For this review, take the finished solid that the model builds, in its own axes (mm). A direction names the side the tool comes from. Coordinates: 2 decimals unless noted, no trailing zeros. Loops run counter-clockwise (first coordinate to the right, second up) from the corner with the lowest first, then second, coordinate; pieces in that order, holes last. Notation, with made-up numbers: M 20,9 L 63,9 A20 ccw 63,41 Z; hole C 14.5,31 d9. An arc over 180 degrees is marked long. Write each question's results on one line, items separated by ' | '. Start each with the question number.
```python
from build123d import *

# Parameters (mm, degrees)
SKETCH1_R           = 80
BOSS_EXTRUDE1_DEPTH = 3.5
SKETCH2_R           = 10
CUT_EXTRUDE1_DEPTH  = 3.5
BOSS_EXTRUDE2_START = 10
SKETCH3_R           = 30
SKETCH3_R_2         = 10
BOSS_EXTRUDE2_DEPTH = 10
CUT_EXTRUDE2_DEPTH  = 3.5


with BuildPart() as part:
    # Sketch1 → Boss-Extrude1 (new body)
    with BuildSketch(Plane.XY):
        Circle(SKETCH1_R)
    extrude(amount=BOSS_EXTRUDE1_DEPTH)

    # Sketch2 → Cut-Extrude1 (cut)
    with BuildSketch(Plane.XY.offset(3.5)):
        Circle(SKETCH2_R)
    extrude(amount=-CUT_EXTRUDE1_DEPTH, mode=Mode.SUBTRACT)

    # Sketch3 → Boss-Extrude2 (add)
    with BuildSketch(Plane.XY.offset(3.5).offset(BOSS_EXTRUDE2_START)):
        Circle(SKETCH3_R)
        Circle(SKETCH3_R_2, mode=Mode.SUBTRACT)
    extrude(amount=-BOSS_EXTRUDE2_DEPTH)

    # Sketch6 → Cut-Extrude2 (cut)
    with BuildSketch(Plane.XY.offset(3.5)):
        with BuildLine():
            Line((36.837168574, 28.196152423), (51.559600438, 36.696152423))
            ThreePointArc((51.559600438, 36.696152423), (59.755752861, 34.5), (57.559600438, 26.303847577))
            Line((57.559600438, 26.303847577), (42.837168574, 17.803847577))
            ThreePointArc((42.837168574, 17.803847577), (34.641016151, 20), (36.837168574, 28.196152423))
        make_face()
        with BuildLine():
            Line((42.837168574, -17.803847577), (57.559600438, -26.303847577))
            ThreePointArc((57.559600438, -26.303847577), (59.755752861, -34.5), (51.559600438, -36.696152423))
            Line((51.559600438, -36.696152423), (36.837168574, -28.196152423))
            ThreePointArc((36.837168574, -28.196152423), (34.641016151, -20), (42.837168574, -17.803847577))
        make_face()
        with BuildLine():
            Line((6, -46), (6, -63))
            ThreePointArc((6, -63), (0, -69), (-6, -63))
            Line((-6, -63), (-6, -46))
            ThreePointArc((-6, -46), (0, -40), (6, -46))
        make_face()
        with BuildLine():
            Line((-36.837168574, -28.196152423), (-51.559600438, -36.696152423))
            ThreePointArc((-51.559600438, -36.696152423), (-59.755752861, -34.5), (-57.559600438, -26.303847577))
            Line((-57.559600438, -26.303847577), (-42.837168574, -17.803847577))
            ThreePointArc((-42.837168574, -17.803847577), (-34.641016151, -20), (-36.837168574, -28.196152423))
        make_face()
        with BuildLine():
            Line((-42.837168574, 17.803847577), (-57.559600438, 26.303847577))
            ThreePointArc((-57.559600438, 26.303847577), (-59.755752861, 34.5), (-51.559600438, 36.696152423))
            Line((-51.559600438, 36.696152423), (-36.837168574, 28.196152423))
            ThreePointArc((-36.837168574, 28.196152423), (-34.641016151, 20), (-42.837168574, 17.803847577))
        make_face()
        with BuildLine():
            Line((-6, 46), (-6, 63))
            ThreePointArc((-6, 63), (0, 69), (6, 63))
            Line((6, 63), (6, 46))
            ThreePointArc((6, 46), (0, 40), (-6, 46))
        make_face()
    extrude(amount=-CUT_EXTRUDE2_DEPTH, mode=Mode.SUBTRACT)


solid = part.part
```
Q1. Insertion check: P1, Ø3, axis at y = -56, z = 1, coming from the +X side; P2, Ø1.8, axis at y = 52.5, z = 1, coming from the -X side; P3, Ø4, axis at x = -45.5, y = -13, coming from the +Z side. Each pin has a flat end and moves straight along its axis. Give the tip position at first contact, or say it passes through.
Q2. The part is to be moulded in two halves that separate along Y. For faces 1 (the face through (34, 1, 3.5)), 2 (the face through (50.301, 22.113, 1.774)), 3 (the face through (-17.34, -78.1, 1.73)), say which applies: pulls with the +Y half, pulls with the -Y half, needs draft (parallel to the pull), parting line crosses it, or undercut.
Q3. To check wall thickness, follow line 1 along Y through (x, z) = (0, 4); line 2 along Y through (x, z) = (-5, 3); line 3 along Z through (x, y) = (-39, 46). State the ranges of each line that lie inside material, in increasing order.
Q4. Take a section at B-B, the plane x = -0.5. Give the boundary of the cut face in (y, z).
Q5. Take a section at D-D, the plane x = 46.5. Give the boundary of the cut face in (y, z) (3 decimals), then the cut area to 3 significant figures.
Q6. Take a section at C-C, the plane y = 23. Give the boundary of the cut face in (x, z).
Q7. For faces 4 (the face through (-29.97, 1.32, 8.57)), 5 (the face through (13, 0, 13.5)), 6 (the face through (-6, 54, 2)), list the 3-axis set-ups (+Z, -Z, +X, -X, +Y, -Y) from which the entire face can be reached by the end or side of a thin tool; tool diameter is ignored.
Q8. Take a section at A-A, the plane y = 0. Give the boundary of the cut face in (x, z).
Results:
1) P1: x = 58.56 | P2: x = -61.13 | P3: z = 3.5
2) face 1: needs draft | face 2: undercut | face 3: parting line crosses it
3) line 1: -30 to -10, 10 to 30 | line 2: -79.84 to -66.32, -42.68 to -8.66, 8.66 to 42.68, 66.32 to 79.84 | line 3: 0 to 3.5
4) outline: M -80,0 L -68.98,0 L -68.98,3.5 L -80,3.5 Z; M -40.02,0 L -9.99,0 L -9.99,13.5 L -30,13.5 L -30,3.5 L -40.02,3.5 Z; M 9.99,0 L 40.02,0 L 40.02,3.5 L 30,3.5 L 30,13.5 L 9.99,13.5 Z; M 68.98,0 L 80,0 L 80,3.5 L 68.98,3.5 Z
5) outline: M -65.098,0 L -33.775,0 L -33.775,3.5 L -65.098,3.5 Z; M -19.919,0 L 19.919,0 L 19.919,3.5 L -19.919,3.5 Z; M 33.775,0 L 65.098,0 L 65.098,3.5 L 33.775,3.5 Z | area: 359 mm^2
6) outline: M -76.62,0 L -51.84,0 L -51.84,3.5 L -76.62,3.5 Z; M -33.84,0 L 33.84,0 L 33.84,3.5 L 19.26,3.5 L 19.26,13.5 L -19.26,13.5 L -19.26,3.5 L -33.84,3.5 Z; M 51.84,0 L 76.62,0 L 76.62,3.5 L 51.84,3.5 Z
7) face 4: +Z | face 5: +Z, +X, -X, +Y, -Y | face 6: +Z, -Z
8) outline: M -80,0 L -10,0 L -10,13.5 L -30,13.5 L -30,3.5 L -80,3.5 Z; M 10,0 L 80,0 L 80,3.5 L 30,3.5 L 30,13.5 L 10,13.5 Z
